The model under review builds one solid part; all positions refer to its coordinate system, in mm. Face numbers are marked on the shaded views. A direction names the side the tool comes from. Round coordinates to 2 decimals unless told otherwise and drop trailing zeros. Order: outer loops, then holes, each group sorted by start corner. A loop starts at its lowest first (then second) coordinate and runs counter-clockwise, first axis right, second up. Notation, with made-up numbers: (16, -10) -> (32, -10) arc R18 cw to (32, 25) -> close; hole circle Ø4 at (84.5, -40). An arc over 180 degrees is marked (long way). Use a Markdown table: item, result. Add a question column.
```python
from build123d import *

# Parameters (mm, degrees)
ESQUISSE1_R        = 32.5
ESQUISSE1_R_2      = 3.25
BOSS_EXTRU_1_DEPTH = 20
ESQUISSE2_R        = 32
BOSS_EXTRU_2_DEPTH = 150
CONG_1_R           = 20


with BuildPart() as part:
    # Esquisse1 → Boss.-Extru.1 (new body)
    with BuildSketch(Plane(origin=(0, 0, 0), x_dir=(1, 0, 0), z_dir=(0, 1, 0))):
        Circle(ESQUISSE1_R)
        Circle(ESQUISSE1_R_2, mode=Mode.SUBTRACT)
    extrude(amount=BOSS_EXTRU_1_DEPTH)

    # Esquisse2 → Boss.-Extru.2 (add)
    with BuildSketch(Plane(origin=(0, 20, 0), x_dir=(1, 0, 0), z_dir=(0, 1, 0))):
        Circle(ESQUISSE2_R)
    extrude(amount=BOSS_EXTRU_2_DEPTH)

    # Congé1
    cong_1_edges = [part.edges().sort_by_distance(p)[0] for p in [
        (-32, 170, 0),
    ]]
    fillet(cong_1_edges, radius=CONG_1_R)


solid = part.part
```
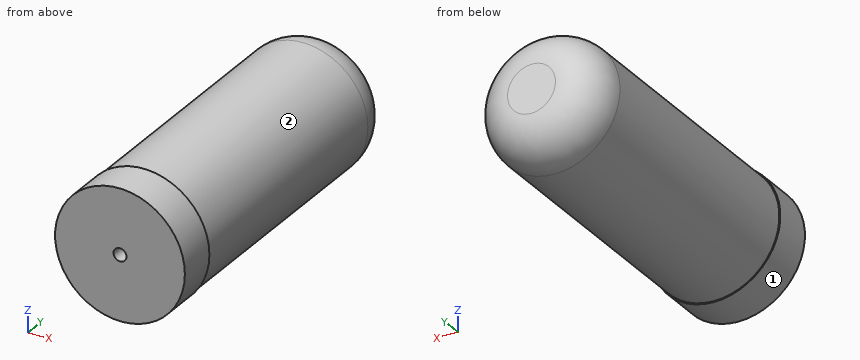
Q1. Add section A-A, the plane y = 137. Give the boundary of the cut face in (x, z).
Q2. For pin 1 (10 mm diameter, centred on y = 98.5, z = 11.5, fed in from -X); pin 2 (8 mm diameter, centred on x = 20.5, y = 56.5, fed in from -Z); pin 3 (2 mm diameter, centred on x = 4, y = 30, fed in from -Z), all flat-tipped, find the tip position at first contact; note any pin that passes through.
Q3. To check wall thickness, follow line 1 along X through (y, z) = (7.5, 0); line 2 along Y through (x, z) = (7.5, -17.5). State the ranges of each line that lie inside material, in increasing order.
Q4. For the marked faces 1 and 2, list the 3-axis set-ups (+Z, -Z, +X, -X, +Y, -Y) from which the entire face can be reached by the end or side of a thin tool; tool diameter is ignored.
Return value:
| question | item | result |
|---|---|---|
| 1 | outline | circle Ø64 at (0, 0) |
| 2 | pin 1 | x = -31.33 |
| 2 | pin 2 | z = -27.42 |
| 2 | pin 3 | z = -31.86 |
| 3 | line 1 | -32.5 to -3.25, 3.25 to 32.5 |
| 3 | line 2 | 0 to 168.72 |
| 4 | face 1 | +Y, -Y |
| 4 | face 2 | +Y |
